Could you check a few things on this model? Use its own coordinates, in mm. Face numbers are marked on the shaded views. A direction names the side the tool comes from. Coordinates: 2 decimals unless noted, no trailing zeros. Loops run counter-clockwise (first coordinate to the right, second up) from the corner with the lowest first, then second, coordinate; pieces in that order, holes last.
1) Imagine slicing it at A-A on z = -6.5. Please give me the cut outline in (x, y), plus the area to 3 significant figures.
2) For the marked faces 4 and 5, which set-ups out of +Z, -Z, +X, -X, +Y, -Y let a thin tool reach every point of the face, with its end or its side?
3) Will these pins go through, and if not, where does the flat tip stop? P1, Ø20, axis at y = 12, z = -11, coming from the +X side; P2, Ø6, axis at y = 15.5, z = 41.5, coming from the +X side.
4) Imagine slicing it at B-B on x = -24.5. Please give me the cut outline in (y, z).
5) Imagine slicing it at C-C on y = 19. Please give me the cut outline in (x, z), plus the area to 3 significant figures.
6) Thinking about a two-plate mould opening in Z: for the marked faces 1, 2 and 3, which applies, released by +Z, released by -Z, zero draft, split by the parting line, or undercut?
7) If I drill on line 1 along Z through (x, y) = (-45.5, 4); line 2 along X through (y, z) = (19, 1); line 3 along X through (y, z) = (12.5, 45), over which ranges is the centre line in solid material (lowest first)?
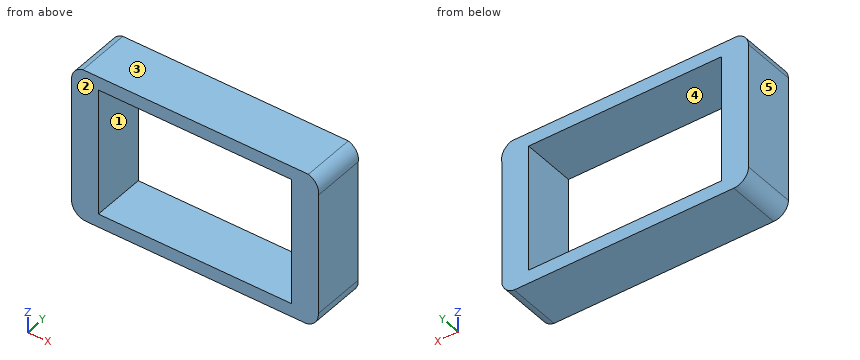
```python
from build123d import *

# Parameters (mm, degrees)
SKETCH1_W           = 144.077216911
SKETCH1_H           = 95
BOSS_EXTRUDE1_DEPTH = 40
SKETCH1_2_W         = 144.077216911
SKETCH1_2_H         = 95
BOSS_EXTRUDE2_DEPTH = 40


with BuildPart() as part:
    # Sketch1 → Boss-Extrude1 (new body)
    with BuildSketch(Plane(origin=(0, 0, 0), x_dir=(1, 0, 0), z_dir=(0, 1, 0))):
        with BuildLine():
            Line((82.709021157, -55.64828922), (-85.557066869, -55.64828922))
            ThreePointArc((-85.557066869, -55.64828922), (-91.537525449, -51.905150215), (-94.013859445, -45.298733306))
            Line((-94.013859445, -45.298733306), (-94.013859445, 48.380180377))
            ThreePointArc((-94.013859445, 48.380180377), (-90.771939739, 56.150001197), (-82.985463341, 59.35171078))
            Line((-82.985463341, 59.35171078), (80.864804877, 59.35171078))
            ThreePointArc((80.864804877, 59.35171078), (87.782044869, 55.253574592), (90.063357466, 47.543935031))
            Line((90.063357466, 47.543935031), (90.063357466, -43.073295521))
            ThreePointArc((90.063357466, -43.073295521), (88.766131999, -50.752673698), (82.709021157, -55.64828922))
        make_face()
        with Locations((-1.97525099, 1.85171078)):
            Rectangle(SKETCH1_W, SKETCH1_H, mode=Mode.SUBTRACT)
    extrude(amount=BOSS_EXTRUDE1_DEPTH)

    # Sketch1<2> → Boss-Extrude2 (add)
    with BuildSketch(Plane(origin=(0, 0, 0), x_dir=(1, 0, 0), z_dir=(0, 1, 0))):
        with BuildLine():
            Line((82.709021157, -55.64828922), (-85.557066869, -55.64828922))
            ThreePointArc((-85.557066869, -55.64828922), (-91.537525449, -51.905150215), (-94.013859445, -45.298733306))
            Line((-94.013859445, -45.298733306), (-94.013859445, 48.380180377))
            ThreePointArc((-94.013859445, 48.380180377), (-90.771939739, 56.150001197), (-82.985463341, 59.35171078))
            Line((-82.985463341, 59.35171078), (80.864804877, 59.35171078))
            ThreePointArc((80.864804877, 59.35171078), (87.782044869, 55.253574592), (90.063357466, 47.543935031))
            Line((90.063357466, 47.543935031), (90.063357466, -43.073295521))
            ThreePointArc((90.063357466, -43.073295521), (88.766131999, -50.752673698), (82.709021157, -55.64828922))
        make_face()
        with Locations((-1.97525099, 1.85171078)):
            Rectangle(SKETCH1_2_W, SKETCH1_2_H, mode=Mode.SUBTRACT)
    extrude(amount=BOSS_EXTRUDE2_DEPTH)


solid = part.part
```
Filled in:
1. outline: (-94.01, 0) - (-74.01, 0) - (-74.01, 40) - (-94.01, 40) - close; (70.06, 0) - (90.06, 0) - (90.06, 40) - (70.06, 40) - close
1. area: 1,600 mm2
2. face 4: +Y, -Y
2. face 5: +Z, -Z, -X, +Y, -Y
3. P1: stops at x = 90.06
3. P2: stops at x = 90.25
4. outline: (0, -59.35) - (40, -59.35) - (40, -49.35) - (0, -49.35) - close; (0, 45.65) - (40, 45.65) - (40, 55.65) - (0, 55.65) - close
5. outline: (-94.01, -48.38) arc R11 ccw to (-82.99, -59.35) - (80.86, -59.35) arc R11 ccw to (90.06, -47.54) - (90.06, 43.07) arc R11 ccw to (82.71, 55.65) - (-85.56, 55.65) arc R11 ccw to (-94.01, 45.3) - close; hole (-74.01, -49.35) - (70.06, -49.35) - (70.06, 45.65) - (-74.01, 45.65) - close
5. area: 7,390 mm2
6. face 1: undercut
6. face 2: zero draft
6. face 3: released by +Z
7. line 1: z = -59.35 to -49.35, 45.65 to 55.65
7. line 2: x = -94.01 to -74.01, 70.06 to 90.06
7. line 3: x = -94.01 to -74.01, 70.06 to 90.27
